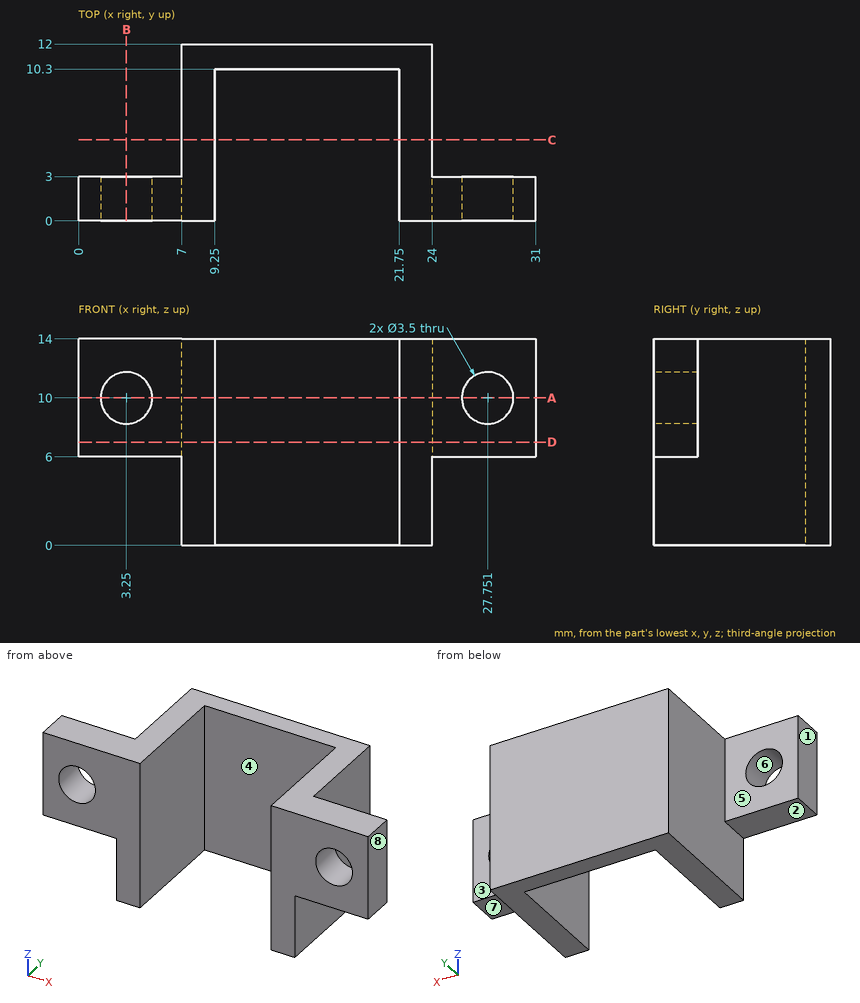
Answer from the drawing. Dimensions are ordinates in mm from the lowest x, y and z of the part. A direction names the side the tool comes from. Give positions to 0.01 mm unless a question says otherwise; leave off trailing zeros. Write each loop counter-clockwise with the first axis right and the second up, starting at its lowest first coordinate (ties: lowest second). Pieces come first, ordered by that corner, then holes.
1) Find the intervals of material crossed by L1, parallel to X at y = 1.25, z = 12.5; L2, parallel to X at y = 7.5, z = 11.25; L3, parallel to Z at x = 3.25, y = 2.1, in increasing order.
2) Section B-B (x = 3.25) is taken. Write down the section's boundary in (y, z).
3) Section A-A (z = 10) is taken. Write down the section's boundary in (x, y).
4) Given P1, Ø0.9, axis at x = 26.5, y = 2, coming from the -Z side; P2, Ø4.5, axis at x = 27.75, z = 10, coming from the +Y side; P3, Ø3, axis at y = 9, z = 4, coming from the -X side, each flat-ended and moving along its own axis, determine where each tip first touches the part or whether it passes through.
5) Section D-D (z = 7) is taken. Write down the section's boundary in (x, y), and give its area (3 significant figures).
6) A tool of negligible diameter and unlimited length cuts with its end or side. For the marked faces 1, 2, 3, 4 and 5, from which of +Z, -Z, +X, -X, +Y, -Y can it reach the whole face along a straight path? Write none if from no direction.
7) For a pull along X with two mould halves and no side action, classify the marked faces 6, 7 and 8 as pulls with the +X half, pulls with the -X half, needs draft (parallel to the pull), parting line crosses it, or undercut.
8) Section C-C (y = 5.5) is taken. Write down the section's boundary in (x, z).
Response:
1. L1: x = 0 to 9.25, 21.75 to 31
1. L2: x = 7 to 9.25, 21.75 to 24
1. L3: z = 6 to 8.25, 11.75 to 14
2. outline: (0, 6) - (3, 6) - (3, 8.25) - (0, 8.25) - close; (0, 11.75) - (3, 11.75) - (3, 14) - (0, 14) - close
3. outline: (0, 0) - (1.5, 0) - (1.5, 3) - (0, 3) - close; (5, 0) - (9.25, 0) - (9.25, 10.3) - (21.75, 10.3) - (21.75, 0) - (26, 0) - (26, 3) - (24, 3) - (24, 12) - (7, 12) - (7, 3) - (5, 3) - close; (29.5, 0) - (31, 0) - (31, 3) - (29.5, 3) - close
4. P1: stops at z = 6
4. P2: stops at y = 3
4. P3: stops at x = 7
5. outline: (0, 0) - (9.25, 0) - (9.25, 10.3) - (21.75, 10.3) - (21.75, 0) - (31, 0) - (31, 3) - (24, 3) - (24, 12) - (7, 12) - (7, 3) - (0, 3) - close
5. area: 117 mm2
6. face 1: +Z, -Z, -X, +Y, -Y
6. face 2: -Z, -X, +Y, -Y
6. face 3: +Z, -Z, +X, +Y
6. face 4: +Z, -Z, -Y
6. face 5: +Z, -Z, -X, +Y
7. face 6: undercut
7. face 7: needs draft
7. face 8: pulls with the +X half
8. outline: (7, 0) - (9.25, 0) - (9.25, 14) - (7, 14) - close; (21.75, 0) - (24, 0) - (24, 14) - (21.75, 14) - close
